```python
from build123d import *

# Parameters (mm, degrees)
F0_W     = 88.2
F0_H     = 73.2
F1_DEPTH = 1.2
F2_W     = 88.2
F2_H     = 73.2
F2_W_2   = 85.8
F2_H_2   = 70.8
F3_DEPTH = 30
F5_DEPTH = 5


with BuildPart() as f1:
    # F0 (on Top) → F1 (new body)
    with BuildSketch(Plane.XY):
        Rectangle(F0_W, F0_H)
    extrude(amount=F1_DEPTH)

    # F2 (on face) → F3 (join)
    with BuildSketch(Plane.XY.offset(1.2)):
        Rectangle(F2_W, F2_H)
        Rectangle(F2_W_2, F2_H_2, mode=Mode.SUBTRACT)
    extrude(amount=F3_DEPTH)

    # F4 (on face) → F5 (join)
    with BuildSketch(Plane.XY.offset(31.2)):
        Polygon((39.1, -36.6), (44.1, -36.6), (44.1, -35.4), (44.1, -31.6), (42.9, -31.6), (42.9, -35.4), (39.1, -35.4), align=None)
        Polygon((42.9, 31.6), (44.1, 31.6), (44.1, 35.4), (44.1, 36.6), (39.1, 36.6), (39.1, 35.4), (42.9, 35.4), align=None)
        Polygon((-44.1, 35.4), (-44.1, 31.6), (-42.9, 31.6), (-42.9, 35.4), (-39.1, 35.4), (-39.1, 36.6), (-44.1, 36.6), align=None)
    extrude(amount=F5_DEPTH)


solid = f1.part
```
Input: part model. Units: mm. Frame: model coordinates. A direction names the side the tool comes from. Give positions to 0.01 mm unless a question says otherwise; leave off trailing zeros. Order: outer loops, then holes, each group sorted by start corner. A loop starts at its lowest first (then second) coordinate and runs counter-clockwise, first axis right, second up. Notation, with made-up numbers: (87.25, 86) - (141.25, 86) arc R20 ccw to (141.25, 93) - close; hole circle Ø6 at (3, 15). An arc over 180 degrees is marked (long way). Use a Markdown table: item, result.
(1) Section query C-C (x = 33.5). Output: boundary loops of the cut face in (y, z).
Computed values:
| item | result |
|---|---|
| outline | (-36.6, 0) - (36.6, 0) - (36.6, 31.2) - (35.4, 31.2) - (35.4, 1.2) - (-35.4, 1.2) - (-35.4, 31.2) - (-36.6, 31.2) - close |
(2) Draft query along X for faces 3 (the flat face through (1, -35.4, 15)), 4 (the flat face through (43.2, 35.2, 36.2)), 5 (the flat face through (-44.1, -1, 18)). Return one class per face: released by +X, released by -X, zero draft, split by the parting line, or undercut.
Computed values:
| item | result |
|---|---|
| face 3 | undercut |
| face 4 | zero draft |
| face 5 | released by -X |
(3) Line query: line 1 (Y direction, x = 20, z = 8); line 2 (X direction, y = 2, z = 18.5); line 3 (Z direction, x = -1, y = -33). Output: solid intervals per line, ascending. Write a range as from..to.
Computed values:
| item | result |
|---|---|
| line 1 | y = -36.6..-35.4, 35.4..36.6 |
| line 2 | x = -44.1..-42.9, 42.9..44.1 |
| line 3 | z = 0..1.2 |
(4) Pin query (flat end, axial travel): pin 1 (1.3 mm diameter, centred on x = 43.5, y = -6, fed in from +Z); pin 2 (1 mm diameter, centred on y = -36, z = 33, fed in from -X); pin 3 (5 mm diameter, centred on x = 9.5, y = -16.5, fed in from +Z). Return the tip coordinate at first contact, or that it passes through.
Computed values:
| item | result |
|---|---|
| pin 1 | stops at z = 31.2 |
| pin 2 | stops at x = 39.1 |
| pin 3 | stops at z = 1.2 |
(5) Section query A-A (z = 27.5). Output: boundary loops of the cut face in (x, y).
Computed values:
| item | result |
|---|---|
| outline | (-44.1, -36.6) - (44.1, -36.6) - (44.1, 36.6) - (-44.1, 36.6) - close; hole (-42.9, -35.4) - (42.9, -35.4) - (42.9, 35.4) - (-42.9, 35.4) - close |
(6) Section query B-B (y = 18). Output: boundary loops of the cut face in (x, z), then the cut area to 3 significant figures.
Computed values:
| item | result |
|---|---|
| outline | (-44.1, 0) - (44.1, 0) - (44.1, 31.2) - (42.9, 31.2) - (42.9, 1.2) - (-42.9, 1.2) - (-42.9, 31.2) - (-44.1, 31.2) - close |
| area | 178 mm2 |
(7) Access query for faces 1 (the flat face through (42.9, 0, 18)), 2 (the flat face through (44.1, -1, 18)). Directions: +Z, -Z, +X, -X, +Y, -Y. A direction counts if a zero-diameter tool reaches every point of the face in a straight line with its end or side. Return the directions, or none.
Computed values:
| item | result |
|---|---|
| face 1 | +Z |
| face 2 | +Z, -Z, +X, +Y, -Y |
